from build123d import *

# Parameters (mm, degrees)
F1_DEPTH = 25.4


with BuildPart() as f1:
    # F0 (on Right) → F1 (new body)
    with BuildSketch(Plane.YZ):
        with BuildLine():
            Line((-3.81, 22.86), (-3.81, 25.112624))
            ThreePointArc((-3.81, 25.112624), (0, -25.4), (3.81, 25.112624))
            Line((3.81, 25.112624), (3.81, 22.86))
            Line((3.81, 22.86), (-3.81, 22.86))
        make_face()
        with BuildLine():
            ThreePointArc((-5.679613, -5.08), (0, 7.62), (5.679613, -5.08))
            Line((5.679613, -5.08), (-5.679613, -5.08))
        make_face(mode=Mode.SUBTRACT)
    extrude(amount=F1_DEPTH)


solid = f1.part
Input: part model. Units: mm. Frame: model coordinates. A direction names the side the tool comes from. Coordinates: 2 decimals unless noted, no trailing zeros. Loops run counter-clockwise (first coordinate to the right, second up) from the corner with the lowest first, then second, coordinate; pieces in that order, holes last. Notation, with made-up numbers: (-0.75, -24) - (56.25, -24) arc R23 cw to (56.25, -9) - close; hole circle Ø7 at (40, 17.25). An arc over 180 degrees is marked (long way). Answer in a Markdown table with one row per item. Add a question column.
Item 1: Section query B-B on z = 0. Return the cut outline in (x, y).
Item 2: Line query: line 1 along Y through (x, z) = (5.5, 0); line 2 along Z through (x, y) = (6.75, -1); line 3 along Z through (x, y) = (24.25, 1.5). Output: solid intervals per line, ascending. Write a range as [from, to].
Item 3: Section query C-C on x = 23.5. Return the cut outline in (y, z), then the cut area to 3 significant figures.
Item 4: Access query for faces 1 (the flat face through (13, 3.81, 24)), 2 (the flat face through (0, -0.4, -5.4)). Directions: +Z, -Z, +X, -X, +Y, -Y. A direction counts if a zero-diameter tool reaches every point of the face in a straight line with its end or side. Return the directions, or none.
Item 5: Section query D-D on z = 11. Return the cut outline in (x, y), then the cut area to 3 significant figures.
Item 6: Contact query for flat-ended pins moving along their axis: P1, Ø1.1, axis at x = 18.5, z = 24, coming from the +Y side; P2, Ø13.5, axis at y = 0, z = 0, coming from the +X side; P3, Ø9, axis at x = 10, y = -2, coming from the +Z side; P4, Ø1.8, axis at x = 18, z = 24, coming from the -Y side. Output: stop coordinate, or through.
Item 7: Section query A-A on y = 0. Return the cut outline in (x, z).
Item 8: Mould query, pull axis Y, two halves, no side actions, for faces 3 (the cylindrical face through (12.522, -1.063, -25.378)), 4 (the flat face through (25.4, -0.4, -5.4)), 5 (the flat face through (13, 0, -5.08)). Classes: released by +Y, released by -Y, zero draft, split by the parting line, or undercut.
Recorded:
| question | item | result |
|---|---|---|
| 1 | outline | (0, -25.4) - (25.4, -25.4) - (25.4, -7.62) - (0, -7.62) - close; (0, 7.62) - (25.4, 7.62) - (25.4, 25.4) - (0, 25.4) - close |
| 2 | line 1 | [-25.4, -7.62], [7.62, 25.4] |
| 2 | line 2 | [-25.38, -5.08], [7.55, 22.86] |
| 2 | line 3 | [-25.36, -5.08], [7.47, 22.86] |
| 3 | outline | (-3.81, 22.86) - (-3.81, 25.11) arc R25.4 ccw (long way) to (3.81, 25.11) - (3.81, 22.86) - close; hole (-5.68, -5.08) - (5.68, -5.08) arc R7.62 ccw (long way) to start |
| 3 | area | 1,850 mm^2 |
| 4 | face 1 | +Z, +X, -X |
| 4 | face 2 | +Z, -Z, -X, +Y, -Y |
| 5 | outline | (0, -22.89) - (25.4, -22.89) - (25.4, 22.89) - (0, 22.89) - close |
| 5 | area | 1,160 mm^2 |
| 6 | P1 | y = 9.76 |
| 6 | P2 | x = 25.4 |
| 6 | P3 | z = 25.11 |
| 6 | P4 | y = -10.56 |
| 7 | outline | (0, -25.4) - (25.4, -25.4) - (25.4, -5.08) - (0, -5.08) - close; (0, 7.62) - (25.4, 7.62) - (25.4, 22.86) - (0, 22.86) - close |
| 8 | face 3 | split by the parting line |
| 8 | face 4 | zero draft |
| 8 | face 5 | undercut |
